Could you check a few things on this drawing? It's one solid part, dimensions in mm from its lowest x, y, z. Coordinates: 2 decimals unless noted, no trailing zeros. Write each loop counter-clockwise with the first axis right and the second up, starting at its lowest first coordinate (ties: lowest second). Pieces come first, ordered by that corner, then holes. Notation, with made-up numbers: (66.5, 63) - (117.5, 63) arc R11 cw to (117.5, 77) - close; hole circle Ø10 at (-15, -23). An arc over 180 degrees is marked (long way). Answer as a JSON object with one key per item and string values. Group by question number.
1) Please list where these lines run through material, in increasing order: line 1 along Z through (x, y) = (87.5, 14) (1 decimal); line 2 along Y through (x, z) = (63, 89); line 3 along Z through (x, y) = (28.5, 6) (1 decimal).
2) Will these pins go through, and if not, where does the flat tip stop? pin 1 Ø12 at (y, z) = (52.5, 53) entering from +X; pin 2 Ø10 at (x, z) = (27, 34.5) entering from +Y; pin 3 Ø2 at (y, z) = (34.5, 28) entering from -X.
3) If we section it at A-A (x = 53): Write out the boundary of the cut face in (y, z), plus the area to 3 significant figures.
4) If we section it at C-C (z = 88): Write out the boundary of the cut face in (x, y).
5) If we section it at D-D (z = 73): Write out the boundary of the cut face in (x, y).
6) If we section it at B-B (y = 18): Write out the boundary of the cut face in (x, z).
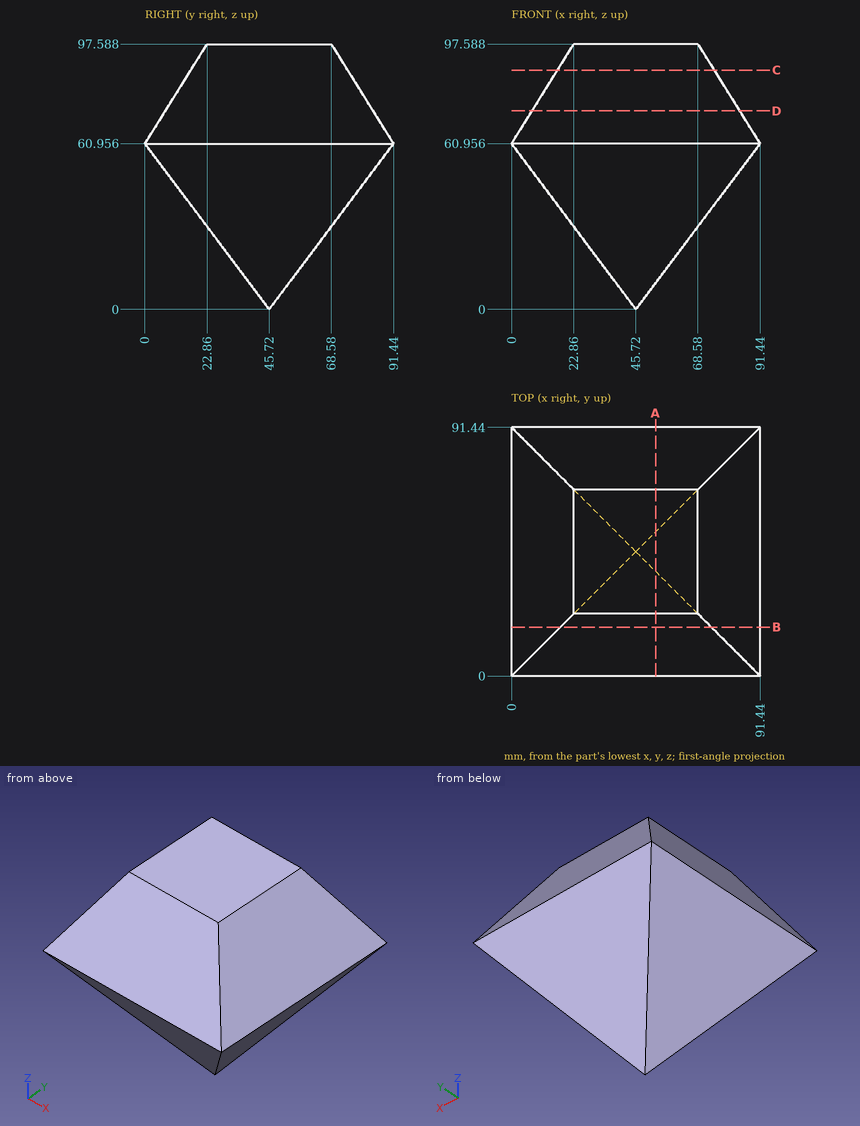
Here are the results:
{
 "1": {"line 1": "z = 55.7 to 67.3", "line 2": "y = 17.5 to 73.94", "line 3": "z = 53 to 70.6"},
 "2": {"pin 1": "stops at x = 89.97", "pin 2": "stops at y = 75.35", "pin 3": "stops at x = 23.97"},
 "3": {"outline": "(0, 60.96) - (38.44, 9.71) - (53, 9.71) - (91.44, 60.96) - (68.58, 97.59) - (22.86, 97.59) - close", "area": "5,230 mm²"},
 "4": {"outline": "(16.88, 16.88) - (74.56, 16.88) - (74.56, 74.56) - (16.88, 74.56) - close"},
 "5": {"outline": "(7.52, 7.52) - (83.92, 7.52) - (83.92, 83.92) - (7.52, 83.92) - close"},
 "6": {"outline": "(0, 60.96) - (18, 36.96) - (73.44, 36.96) - (91.44, 60.96) - (73.44, 89.8) - (18, 89.8) - close"}
}
